Build history of the part. All positions in model axes, mm. A direction names the side the tool comes from. Give positions to 0.01 mm unless a question says otherwise; leave off trailing zeros. Order: outer loops, then holes, each group sorted by start corner. A loop starts at its lowest first (then second) coordinate and runs counter-clockwise, first axis right, second up. Notation, with made-up numbers: (58, 80) - (69, 80) arc R18 ccw to (69, 88) - close; hole circle Ø9 at (7.5, 49.25). An arc over 180 degrees is marked (long way). Write each question's results on one line, items separated by ' | '. Start each with the question number.
1) Drill centre lines: line 1 along Y through (x, z) = (30, -112); line 2 along Z through (x, y) = (18, 78.5); line 3 along Y through (x, z) = (9, -32.5). Where is each one in solid material? Low to high. Write a range as from..to.
2) Cut at A-A on x = 30. List the corners of the cut face in (y, z).
3) Cut at B-B on y = 41. List the corners of the cut face in (x, z), plus the area to 3 significant figures.
4) Tool access for faces 1 (the face through (30, 5, 0)), 2 (the face through (30, 53, -100)): list every direction of +Z, -Z, +X, -X, +Y, -Y with a clear straight run to the whole face (end or side of a thin tool).
5) Cut at D-D on x = 18. List the corners of the cut face in (y, z).
6) Drop flat-ended pins along their axis: pin 1 Ø5 at (x, z) = (36.5, -59) entering from +Y; pin 2 Ø4 at (y, z) = (81.5, -107.5) entering from +X; pin 3 Ø1 at (y, z) = (70.5, -108) entering from -X. Give the stop position or say it passes through.
7) Two-plate mould, pull along Y, no slides. Class faces 3 (the face through (30, 0, -63)), 4 (the face through (31.24, 73.42, -112.68)), 5 (the face through (30, 48, -125)): +Y half, -Y half, draft (parallel to the pull), parting line (faces both ways), or undercut.
8) Cut at C-C on z = -97. List the corners of the cut face in (x, y).
from build123d import *

# Parameters (mm, degrees)
SKETCH1_W           = 60
SKETCH1_H           = 125
BOSS_EXTRUDE1_DEPTH = 10
SKETCH2_R           = 9.5
BOSS_EXTRUDE2_DEPTH = 25


with BuildPart() as part:
    # Sketch1 → Boss-Extrude1 (new body)
    with BuildSketch(Plane(origin=(0, 0, 0), x_dir=(1, 0, 0), z_dir=(0, 1, 0))):
        with Locations((30, 62.5)):
            Rectangle(SKETCH1_W, SKETCH1_H)
    extrude(amount=BOSS_EXTRUDE1_DEPTH)

    # Sketch2 → Boss-Extrude2 (add)
    with BuildSketch(Plane(origin=(0, 0, -125), x_dir=(-1, 0, 0), z_dir=(0, 0, -1))):
        with BuildLine():
            Line((-60, 10), (0, 10))
            Line((0, 10), (0, 64))
            ThreePointArc((0, 64), (-30, 94), (-60, 64))
            Line((-60, 64), (-60, 10))
        make_face()
        with Locations((-30, 64)):
            Circle(SKETCH2_R, mode=Mode.SUBTRACT)
    extrude(amount=-BOSS_EXTRUDE2_DEPTH)


solid = part.part
Results:
1) line 1: 0..54.5, 73.5..94 | line 2: -125..-100 | line 3: 0..10
2) outline: (0, -125) - (54.5, -125) - (54.5, -100) - (10, -100) - (10, 0) - (0, 0) - close; (73.5, -125) - (94, -125) - (94, -100) - (73.5, -100) - close
3) outline: (0, -125) - (60, -125) - (60, -100) - (0, -100) - close | area: 1,500 mm^2
4) face 1: +Z, +X, -X, +Y, -Y | face 2: +Z, +X, -X, +Y
5) outline: (0, -125) - (91.5, -125) - (91.5, -100) - (10, -100) - (10, 0) - (0, 0) - close
6) pin 1: y = 10 | pin 2: x = 55.69 | pin 3: x = 0.61
7) face 3: -Y half | face 4: undercut | face 5: draft
8) outline: (0, 0) - (60, 0) - (60, 10) - (0, 10) - close
